from build123d import *

# Parameters (mm, degrees)
SKETCH1_W           = 31
SKETCH1_H           = 42.5
BOSS_EXTRUDE1_DEPTH = 3
SKETCH2_W           = 37
SKETCH2_H           = 48.5
SKETCH2_W_2         = 31
SKETCH2_H_2         = 42.5
BOSS_EXTRUDE2_DEPTH = 3
CUT_EXTRUDE1_REACH  = 32.648
SKETCH3_R           = 1.65
FILLET4_R           = 1


with BuildPart() as part:
    # Sketch1 → Boss-Extrude1 (new body)
    with BuildSketch(Plane.XY):
        Rectangle(SKETCH1_W, SKETCH1_H)
    extrude(amount=BOSS_EXTRUDE1_DEPTH)

    # Sketch2 → Boss-Extrude2 (add)
    with BuildSketch(Plane.XY):
        Rectangle(SKETCH2_W, SKETCH2_H)
        Rectangle(SKETCH2_W_2, SKETCH2_H_2, mode=Mode.SUBTRACT)
    extrude(amount=BOSS_EXTRUDE2_DEPTH)

    # Sketch3 → Cut-Extrude1 (cut, up to next)
    with BuildSketch(Plane(origin=(0, 0, 0), x_dir=(-1, 0, 0), z_dir=(0, 0, -1)), mode=Mode.PRIVATE) as cut_extrude1_sk1:
        with Locations((12.35, 18.6)):
            Circle(SKETCH3_R)
    cut_extrude1_tool1 = extrude(cut_extrude1_sk1.sketch, amount=-CUT_EXTRUDE1_REACH, mode=Mode.PRIVATE) & part.part
    # Sketch3 → Cut-Extrude1 (cut, up to next)
    with BuildSketch(Plane(origin=(0, 0, 0), x_dir=(-1, 0, 0), z_dir=(0, 0, -1)), mode=Mode.PRIVATE) as cut_extrude1_sk2:
        with Locations((0, -18.6)):
            Circle(SKETCH3_R)
    cut_extrude1_tool2 = extrude(cut_extrude1_sk2.sketch, amount=-CUT_EXTRUDE1_REACH, mode=Mode.PRIVATE) & part.part
    cut_extrude1_1 = cut_extrude1_tool1.solids().sort_by_distance((-12.35, 18.6, 0))[0]
    add(cut_extrude1_1, mode=Mode.SUBTRACT)
    cut_extrude1_2 = cut_extrude1_tool2.solids().sort_by_distance((0, -18.6, 0))[0]
    add(cut_extrude1_2, mode=Mode.SUBTRACT)
    cut_extrude1 = cut_extrude1_1 + cut_extrude1_2  # Cut-Extrude1 as one shape, for the pattern or mirror that repeats it

    # Mirror1: Cut-Extrude1 across plane
    add(cut_extrude1.mirror(Plane(origin=(0, 0, 0), x_dir=(0, 0, 1), z_dir=(1, 0, 0))), mode=Mode.SUBTRACT)

    # Fillet4
    fillet4_edges = [part.edges().sort_by_distance(p)[0] for p in [
        (0, -24.25, 0),
        (-18.5, -24.25, 1.5),
        (18.5, 0, 0),
        (18.5, -24.25, 1.5),
        (0, 24.25, 0),
        (18.5, 24.25, 1.5),
        (-18.5, 0, 0),
        (-18.5, 24.25, 1.5),
    ]]
    fillet(fillet4_edges, radius=FILLET4_R)


solid = part.part
For this review, take the finished solid that the model builds, in its own axes (mm). Give positions to 0.01 mm unless a question says otherwise; leave off trailing zeros. Order: outer loops, then holes, each group sorted by start corner. A loop starts at its lowest first (then second) coordinate and runs counter-clockwise, first axis right, second up. Notation, with made-up numbers: (-26.5, 37.25) - (7.5, 37.25) arc R11 ccw to (7.5, 52.25) - close; hole circle Ø1 at (68.25, 63). An arc over 180 degrees is marked (long way). Answer as a JSON object with one key per item and string values. Group by question number.
Item 1: Take a section at B-B on y = -18.6. Give the boundary of the cut face in (x, z), and give its area (3 significant figures).
Item 2: Take a section at A-A on x = 0. Give the boundary of the cut face in (y, z), and give its area (3 significant figures).
Item 3: Take a section at C-C on z = 0.5. Give the boundary of the cut face in (x, y).
Item 4: Draft analysis for pull direction Y (two halves, no side actions). For faces 1 (the flat face through (0, 0, 3)), 2 (the cylindrical face through (-18.215, -23.949, 2.014)), 3 (the cylindrical face through (-11.99, 16.99, 1.48)), state which applies: pulls with the +Y half, pulls with the -Y half, needs draft (parallel to the pull), parting line crosses it, or undercut.
Item 5: Wall thickness on line 1 along Y through (x, z) = (-12.35, 1.15); line 2 along X through (y, z) = (-18.6, 1.35); line 3 along Y through (x, z) = (0, 1.85): over which ranges is each line inside the solid? List them lowest first.
Reported:
{
 "1": {"outline": "(-18.5, 1) arc R1 ccw to (-17.5, 0) - (-1.65, 0) - (-1.65, 3) - (-18.5, 3) - close; (1.65, 0) - (17.5, 0) arc R1 ccw to (18.5, 1) - (18.5, 3) - (1.65, 3) - close", "area": "101 mm^2"},
 "2": {"outline": "(-24.25, 1) arc R1 ccw to (-23.25, 0) - (-20.25, 0) - (-20.25, 3) - (-24.25, 3) - close; (-16.95, 0) - (23.25, 0) arc R1 ccw to (24.25, 1) - (24.25, 3) - (-16.95, 3) - close", "area": "135 mm^2"},
 "3": {"outline": "(-18.37, -23.25) arc R0.87 ccw to (-17.5, -24.12) - (17.5, -24.12) arc R0.87 ccw to (18.37, -23.25) - (18.37, 23.25) arc R0.87 ccw to (17.5, 24.12) - (-17.5, 24.12) arc R0.87 ccw to (-18.37, 23.25) - close; hole circle Ø3.3 at (-12.35, 18.6); hole circle Ø3.3 at (0, -18.6); hole circle Ø3.3 at (12.35, 18.6)"},
 "4": {"face 1": "needs draft", "face 2": "pulls with the -Y half", "face 3": "undercut"},
 "5": {"line 1": "-24.25 to 16.95, 20.25 to 24.25", "line 2": "-18.5 to -1.65, 1.65 to 18.5", "line 3": "-24.25 to -20.25, -16.95 to 24.25"}
}
